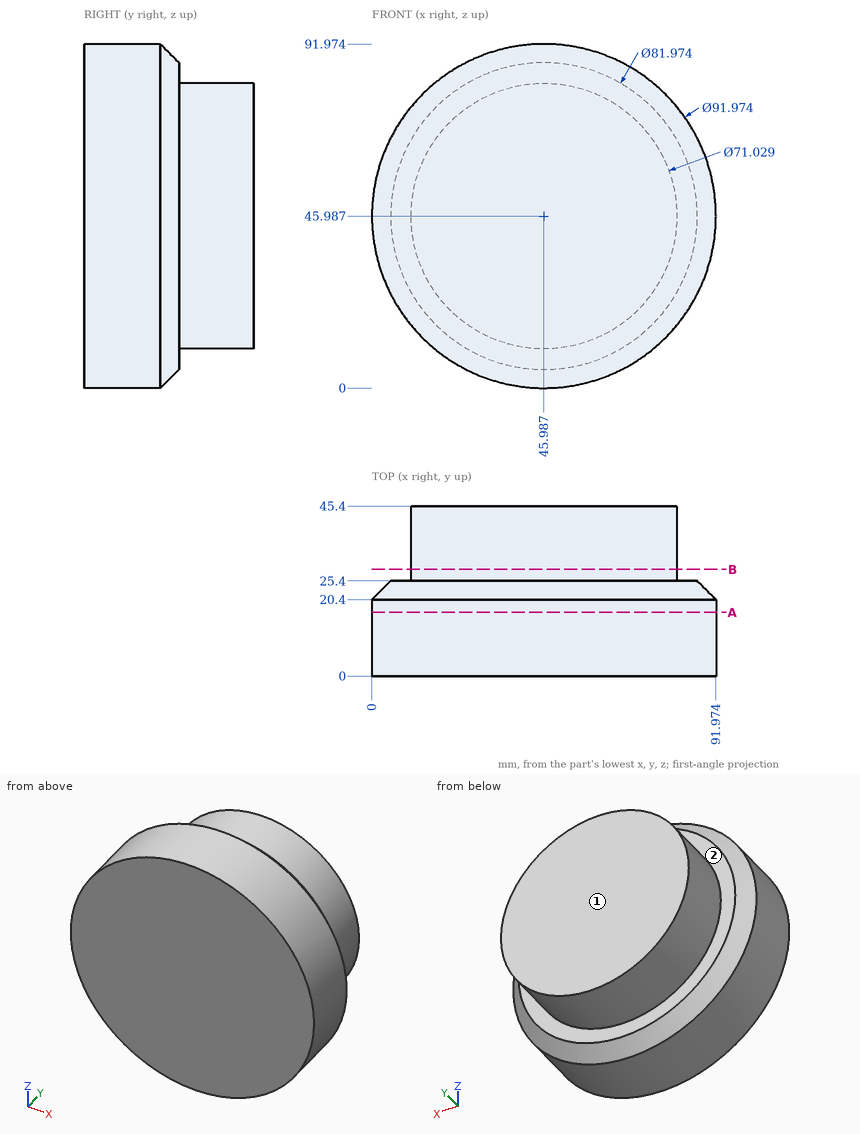
Job drawing, mm, ordinate dimensions from the low corner. One solid piece. A direction names the side the tool comes from. Round coordinates to 2 decimals unless told otherwise and drop trailing zeros. Loops run counter-clockwise (first coordinate to the right, second up) from the corner with the lowest first, then second, coordinate; pieces in that order, holes last. Notation, with made-up numbers: (12.25, 77) -> (17.25, 77) arc R12 cw to (17.25, 90) -> close; hole circle Ø8 at (32, 56.25). An arc over 180 degrees is marked (long way). One line per item, written item: value. Start each with the question number.
Q1. Probe line 1 along X through (y, z) = (38, 47); line 2 along Y through (x, z) = (7.5, 32.5); line 3 along Z through (x, y) = (47, 15.5). List the from-to ranges inside material, lowest first.
Q2. 3-axis set-ups, long thin cutter, end or side, ignore diameter. For the marked faces 1 and 2: which of +Z, -Z, +X, -X, +Y, -Y reach the whole face in a straight line?
Q3. Cut at A-A on y = 17. List the corners of the cut face in (x, z) (1 decimal), plus the area to 3 significant figures.
Q4. Cut at B-B on y = 28.5. List the corners of the cut face in (x, z) (1 decimal), plus the area to 3 significant figures.
Q5. Drop flat-ended pins along their axis: pin 1 Ø8 at (x, y) = (82, 16.5) entering from -Z; pin 2 Ø6 at (y, z) = (8.5, 22) entering from -X; pin 3 Ø1.5 at (y, z) = (12, 33.5) entering from -X. Give the stop position or say it passes through.
Computed:
1. line 1: 10.49 to 81.49
1. line 2: 0 to 25.4
1. line 3: 0.01 to 91.96
2. face 1: +Z, -Z, +X, -X, +Y
2. face 2: +Y
3. outline: circle Ø92 at (46, 46)
3. area: 6,640 mm²
4. outline: circle Ø71 at (46, 46)
4. area: 3,960 mm²
5. pin 1: z = 12.97
5. pin 2: x = 5.07
5. pin 3: x = 1.52
